The listing builds one solid part. Answer for the finished solid, in the listing's coordinates (mm). A direction names the side the tool comes from. Give positions to 0.01 mm unless a question says otherwise; leave off trailing zeros. Write each loop counter-clockwise with the first axis right and the second up, starting at its lowest first coordinate (ties: lowest second). Pieces come first, ordered by that corner, then holes. Notation, with made-up numbers: (46, 38) -> (82, 38) arc R13 cw to (82, 51) -> close; hole circle Ø11 at (-3.5, 12). An arc over 180 degrees is marked (long way). One line per question, with ' | ' between items.
Autodesk Fusion 360 part; units mm, degrees
sketch "Skizze1" plane through (0, 0, 0) normal (0, 0, 1) x (1, 0, 0)
  line L0 (0, 0) -> (39.9, 0) construction
  circle A0 centre (39.9, 0) radius 3.8
  line L1 (33.05, -7.2) -> (46.9, -7.2)
  line L2 (46.9, -7.2) -> (46.9, 42.9968)
  line L3 (45.6, -5.9) -> (45.6, 33.959)
  line L4 (45.6, -5.9) -> (33.05, -5.9)
  line L5 (36.733, 2.1) -> (30.2653, 2.1)
  line L6 (30.2653, 2.1) -> (30.2653, -2.1)
  line L7 (30.2653, -2.1) -> (36.733, -2.1)
  line L8 (36.733, -2.1) -> (36.733, 2.1)
  arc A1 (41.6, -5.9) -> (45.6, -1.9) centre (41.6, -1.9) ccw
  line L9 (43.9, 0) -> (45.4, 0)
  line L10 (45.4, 0) -> (45.4, -1.9)
  arc A2 (36.6274, -2.3) -> (43.9, 0) centre (39.9, 0) ccw
  arc A3 (41.6, -5.7) -> (45.4, -1.9) centre (41.6, -1.9) ccw
  line L11 (41.6, -5.7) -> (32.85, -5.7)
  line L12 (36.6274, -2.3) -> (0, -2.3)
  line L13 (33.05, -7.2) -> (33.05, -5.9)
  line L14 (32.85, -5.7) -> (32.85, -7.3)
  line L15 (32.85, -7.3) -> (35.55, -7.3)
  line L16 (35.55, -7.3) -> (35.55, -8.5)
  line L17 (35.55, -8.5) -> (0, -8.5)
  line L18 (0, -2.3) -> (0, -8.5)
  dimension "d1" = 39.9
  dimension "d2" = 7.6
  dimension "d3" = 7.2
  dimension "d5" = 1.3
  dimension "d6" = 1.3
  dimension "d7" = 4.2
  dimension "d8" = 4
  dimension "d10" = 0.2
  dimension "d11" = 0.2
  dimension "d12" = 0.2
  dimension "d13" = 0.2
  dimension "d14" = 0.2
  dimension "d15" = 33.05
  dimension "d16" = 0.2
  dimension "d17" = 0.1
  dimension "d18" = 2.7
  dimension "d19" = 1.2
  dimension "d47" = 7
extrude "Extrusion1" add sketch "Skizze1" along normal blind 16.4 contours L9 L10 A2 A3 L11 L12 L14 L15 L16 L17 L18
sketch "Skizze2" plane through (0, 0, 0) normal (0, 0, -1) x (1, 0, 0)
  line L0 (0, 2.3) -> (36.6274, 2.3)
  arc A0 (43.9, 0) -> (36.6274, 2.3) centre (39.9, 0) ccw
  line L1 (43.9, 0) -> (45.4, 0)
  line L2 (45.4, 0) -> (45.4, 1.9)
  arc A1 (45.4, 1.9) -> (41.6, 5.7) centre (41.6, 1.9) ccw
  line L3 (41.6, 5.7) -> (32.85, 5.7)
  line L4 (32.85, 5.7) -> (32.85, 7.3)
  line L5 (32.85, 7.3) -> (35.55, 7.3)
  line L6 (35.55, 7.3) -> (35.55, 8.5)
  line L7 (35.55, 8.5) -> (0, 8.5)
  line L8 (0, 8.5) -> (0, 2.3)
  line L9 (32.85, 5.2) -> (32.85, 3)
  line L10 (32.85, 5.2) -> (29.95, 5.2)
  line L11 (29.95, 5.2) -> (29.95, 8.5)
  line L12 (32.85, 3) -> (26.45, 3)
  line L13 (26.45, 3) -> (26.45, 2.3)
  line L14 (32.85, 3) -> (32.85, 2.3) construction
  arc A2 (34.05, 2.3) -> (32.85, 5.2) centre (17.5457, -2.8311) ccw
  dimension "d23" = 3.3
  dimension "d24" = 2.2
  dimension "d25" = 32.85
  dimension "d26" = 2.9
  dimension "d27" = 6.4
  dimension "d34" = 1.2
extrude "Extrusion2" cut sketch "Skizze2" against normal blind 10.8 contours L0 L7 L8 L9 L10 L11 L12 L13
sketch "Skizze3" plane through (0, 0, 10.8) normal (0, 0, -1) x (1, 0, 0)
  line L0 (32.85, 5.2) -> (29.95, 5.2)
  line L1 (29.95, 5.2) -> (29.95, 8.5)
  line L2 (29.95, 8.5) -> (0, 8.5)
  line L3 (0, 8.5) -> (0, 2.3)
  line L4 (0, 2.3) -> (26.45, 2.3)
  line L5 (26.45, 2.3) -> (26.45, 3)
  line L6 (26.45, 3) -> (32.85, 3)
  line L7 (32.85, 3) -> (32.85, 5.2)
  line L8 (29.95, 5.2) -> (0, 5.2)
  line L9 (26.45, 3) -> (0, 3)
extrude "Extrusion3" cut sketch "Skizze3" against normal blind 0.6 contours L0 L3 L6 L7 L8 L9
mirror "Spiegeln1" about plane through (0, 0, 0) normal (1, 0, 0) of bodies 1 merged
extrude "Extrusion4" cut sketch "Skizze2" against normal blind 4.5 contours L0 L9 L12 L13 A2
sketch "Skizze5" plane through (0, 0, 10.8) normal (0, 0, -1) x (1, 0, 0)
  line L0 (26.45, 3) -> (-26.45, 3)
  line L1 (-26.45, 3) -> (-26.45, 2.3)
  line L2 (-26.45, 2.3) -> (26.45, 2.3)
  line L3 (26.45, 2.3) -> (26.45, 3)
  line L4 (-9.5, 2.3) -> (9.5, 2.3)
  line L5 (9.5, 2.3) -> (9.5, 3)
  line L6 (9.5, 3) -> (-9.5, 3)
  line L7 (-9.5, 3) -> (-9.5, 2.3)
  dimension "d39" = 19
extrude "Extrusion6" cut sketch "Skizze5" against normal blind 4.6 contours L0 L2 L4 L5 L6 L7
sketch "Skizze6" plane through (0, 0, 16.4) normal (0, 0, 1) x (-1, 0, 0)
  line L0 (-36.6274, 2.3) -> (36.6274, 2.3)
  arc A0 (43.9, 0) -> (36.6274, 2.3) centre (39.9, 0) ccw
  line L1 (43.9, 0) -> (45.4, 0)
  line L2 (45.4, 0) -> (45.4, 1.9)
  arc A1 (45.4, 1.9) -> (41.6, 5.7) centre (41.6, 1.9) ccw
  line L3 (41.6, 5.7) -> (32.85, 5.7)
  line L4 (32.85, 5.7) -> (32.85, 7.3)
  line L5 (32.85, 7.3) -> (35.55, 7.3)
  line L6 (35.55, 7.3) -> (35.55, 8.5)
  line L7 (35.55, 8.5) -> (-35.55, 8.5)
  line L8 (-35.55, 8.5) -> (-35.55, 7.3)
  line L9 (-35.55, 7.3) -> (-32.85, 7.3)
  line L10 (-32.85, 7.3) -> (-32.85, 5.7)
  line L11 (-32.85, 5.7) -> (-41.6, 5.7)
  arc A2 (-41.6, 5.7) -> (-45.4, 1.9) centre (-41.6, 1.9) ccw
  line L12 (-45.4, 1.9) -> (-45.4, 0)
  line L13 (-45.4, 0) -> (-43.9, 0)
  arc A3 (-36.6274, 2.3) -> (-43.9, 0) centre (-39.9, 0) ccw
  line L14 (32.85, 7.3) -> (-32.85, 7.3)
  line L15 (32.85, 5.7) -> (-32.85, 5.7)
extrude "Extrusion7" cut sketch "Skizze6" against normal blind 3.4 contours L4 L10 L14 L15
extrude "Extrusion8" cut 1 faces at (-12.6469, -4.9624, 16.4) along direction (0, 0, -1) blind 3.4
chamfer "Fase1" distance 0.8 angle 45 3 edges at (35.55, -8.5, 8.2) (0, -8.5, 16.4) (-35.55, -8.5, 8.2)
chamfer "Fase1" distance 0.6 angle 45 2 edges at (9.5, -2.65, 10.8) (-9.5, -2.65, 10.8)
fillet "Abrundung1" radius 2.4 2 edges at (-32.85, -4.1, 11.4) (32.85, -4.1, 11.4)
move_face "Flächen versetzen1" offset 0.5 2 faces at (32.3758, -2.3, 9.4333) (-33.2349, -2.3, 7.9333)
sketch "Skizze7" plane through (0, -1.8, 0) normal (0, 1, 0) x (-1, 0, 0)
  line L0 (9.5, 11.4) -> (10.1, 10.8)
  line L1 (10.1, 10.8) -> (26.45, 10.8)
  line L2 (26.45, 10.8) -> (26.45, 0)
  line L3 (26.45, 0) -> (36.3279, 0)
  line L4 (36.3279, 0) -> (36.3279, 13)
  line L5 (36.3279, 13) -> (9.5, 13)
  line L6 (9.5, 13) -> (9.5, 11.4)
  line L7 (33.9, 13) -> (33.9, 0)
  line L8 (-10.1, 10.8) -> (-9.5, 11.4)
  line L9 (-9.5, 11.4) -> (-9.5, 13)
  line L10 (-9.5, 13) -> (-36.3279, 13)
  line L11 (-36.3279, 13) -> (-36.3279, 0)
  line L12 (-36.3279, 0) -> (-34.1972, 0)
  line L13 (-34.1972, 0) -> (-34.1972, 4.5)
  line L14 (-34.1972, 4.5) -> (-26.45, 4.5)
  line L15 (-26.45, 4.5) -> (-26.45, 10.8)
  line L16 (-26.45, 10.8) -> (-10.1, 10.8)
  line L17 (-33.9, 13) -> (-33.9, 4.5)
  point P0 (43.9, 13)
  point P1 (-43.9, 13)
  dimension "d52" = 10
  dimension "d53" = 10
extrude "Extrusion9" add sketch "Skizze7" along normal blind 1.8 contours L0 L1 L2 L3 L5 L6 L7 | L8 L9 L10 L14 L15 L16 L17
equation "d1 = ( 79.8 / 2 ) * 1 mm"
equation "d3 = 11 mm - ( 7.6 / 2 ) * 1 mm"
equation "toleranz = 0.2 mm"
equation "d10 = toleranz"
equation "d11 = toleranz"
equation "d12 = toleranz"
equation "d13 = toleranz"
equation "d14 = toleranz"
equation "d15 = ( 66.1 / 2 ) * 1 mm"
equation "d16 = toleranz"
equation "d25 = ( 65.7 / 2 ) * 1 mm"
equation "d28 = -10.7 mm + 0.6 mm - 0.7 mm"
equation "d40 = -4.00 mm - 0.6 mm"
Item 1: Flat-ended cylindrical pins translate along their axes: pin 1 (0.5 mm diameter, centred on y = -6.5, z = 8.5, fed in from +X); pin 2 (7 mm diameter, centred on x = 39, z = 7.5, fed in from -Y); pin 3 (0.7 mm diameter, centred on x = 35.5, z = 4.5, fed in from +Y). Find the tip coordinate at first contact, or state that the pin passes through.
Answers below:
pin 1: x = 32.85 | pin 2: y = -7.75 | pin 3: y = -1.8
Item 2: A tool of negligible diameter and unlimited length cuts with its end or side. For faces 1 (the face through (-28, -3, 6)), 2 (the face through (18, -2, 10.8)), 3 (the face through (33.623, -3.512, 2.218)), 4 (the face through (35, -1.8, 6)), from which of +Z, -Z, +X, -X, +Y, -Y can it reach the whole face along a straight path? Write none if from no direction.
Answers below:
face 1: -Z | face 2: -Z, +Y, -Y | face 3: -Z, +Y | face 4: +Z, -Z, +Y
Item 3: Find section C-C (x = 6). Write down the section's boundary in (y, z), then the cut area to 3 significant figures.
Answers below:
outline: (-8.5, 10.8) -> (-5.2, 10.8) -> (-5.2, 11.4) -> (-3, 11.4) -> (-3, 13) -> (-7.3, 13) -> (-7.3, 16.4) -> (-7.7, 16.4) -> (-8.5, 15.6) -> close | area: 14.5 mm²
Item 4: Consider line 1 (Y direction, x = -33.5, z = 4.75); line 2 (Y direction, x = 34.5, z = 11.5); line 3 (X direction, y = -2, z = 3.25). Determine where each line is inside the solid, lowest interval first. Write a range as [from, to].
Answers below:
line 1: [-8.5, -7.3], [-5.7, 0] | line 2: [-8.5, -7.3], [-5.7, -1.8] | line 3: [-45.4, -43.36], [-36.44, -26.45], [34.14, 36.44], [43.36, 45.4]
Item 5: Determine the mould class of faces 5 (the face through (0, -5.2, 11)), 6 (the face through (-1, -4, 13)), 7 (the face through (-45.4, -1, 6)) for opening direction X: pulls with the +X half, pulls with the -X half, needs draft (parallel to the pull), parting line crosses it, or undercut.
Answers below:
face 5: undercut | face 6: needs draft | face 7: pulls with the -X half
Item 6: Find section B-B (x = -17). Write down the section's boundary in (y, z), then the cut area to 3 significant figures.
Answers below:
outline: (-8.5, 10.8) -> (-5.2, 10.8) -> (-5.2, 11.4) -> (-3, 11.4) -> (-3, 10.8) -> (0, 10.8) -> (0, 13) -> (-7.3, 13) -> (-7.3, 16.4) -> (-7.7, 16.4) -> (-8.5, 15.6) -> close | area: 21.1 mm²
Item 7: Find section D-D (x = -38). Write down the section's boundary in (y, z).
Answers below:
outline: (-5.7, 0) -> (-3.52, 0) -> (-3.52, 13) -> (-5.7, 13) -> close
